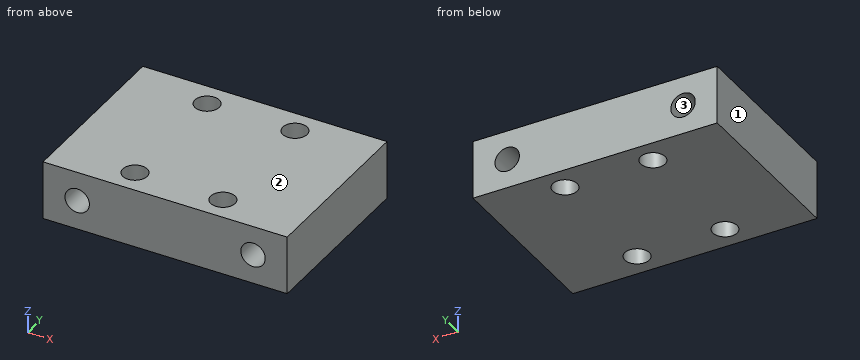
from build123d import *

# Parameters (mm, degrees)
SKETCH_1_W             = 25
SKETCH_1_H             = 18
EXTRUDE_1_DEPTH        = 3
HOLE_WIZARD_M3_1_D     = 2.5
HOLE_WIZARD_M3_2_D     = 2.5
HOLE_WIZARD_M3_2_DEPTH = 8.5
HOLE_WIZARD_M3_2_TIP   = 0.751075774


with BuildPart() as part:
    # 草图1 → 凸台-拉伸1 (new, symmetric)
    with BuildSketch(Plane.XY):
        Rectangle(SKETCH_1_W, SKETCH_1_H)
    extrude(amount=EXTRUDE_1_DEPTH, both=True)

    # M3 螺纹孔1 (through all)
    with Locations(Plane(origin=(0, 9, 0), x_dir=(1, 0, 0), z_dir=(0, 1, 0))):
        with Locations((-9, 0), (9, 0)):
            Hole(HOLE_WIZARD_M3_1_D / 2)

    # M3 螺纹孔2
    with Locations(Plane.XY.offset(3)):
        with Locations((-4.5, -6.5), (4.5, -6.5), (4.5, 6.5), (-4.5, 6.5)):
            Hole(HOLE_WIZARD_M3_2_D / 2, depth=HOLE_WIZARD_M3_2_DEPTH)
            with Locations((0, 0, -(HOLE_WIZARD_M3_2_DEPTH + HOLE_WIZARD_M3_2_TIP / 2))):  # 118° drill point
                Cone(0, HOLE_WIZARD_M3_2_D / 2, HOLE_WIZARD_M3_2_TIP, mode=Mode.SUBTRACT)


solid = part.part
Verification items for the finished model (mm, model axes). Face numbers are marked on the shaded views. Give positions to 0.01 mm unless a question says otherwise; leave off trailing zeros. Write each loop counter-clockwise with the first axis right and the second up, starting at its lowest first coordinate (ties: lowest second). Pieces come first, ordered by that corner, then holes. Notation, with made-up numbers: M 27,61 L 75,61 A14 ccw 75,71 Z; hole C 31.5,58.5 d2. An arc over 180 degrees is marked long. Use CSV: the item, a comma, the result in double quotes.
1) Cross-section at C-C (x = 9). Enter the section's corners in (y, z), plus the area to 3 significant figures.
Final values:
outline,"M -9,-3 L 9,-3 L 9,-1.25 L -9,-1.25 Z; M -9,1.25 L 9,1.25 L 9,3 L -9,3 Z"
area,"63.0 mm²"
2) Cross-section at A-A (y = 6.5). Enter the section's corners in (x, z), plus the area to 3 significant figures.
Final values:
outline,"M -12.5,-3 L -5.75,-3 L -5.75,3 L -12.5,3 Z; M -3.25,-3 L 3.25,-3 L 3.25,3 L -3.25,3 Z; M 5.75,-3 L 12.5,-3 L 12.5,3 L 5.75,3 Z; hole C -9,0 d2.5; hole C 9,0 d2.5"
area,"110 mm²"
3) Cross-section at D-D (y = 2.5). Enter the section's corners in (x, z), plus the area to 3 significant figures.
Final values:
outline,"M -12.5,-3 L 12.5,-3 L 12.5,3 L -12.5,3 Z; hole C -9,0 d2.5; hole C 9,0 d2.5"
area,"140 mm²"
4) Cross-section at B-B (z = -0.75). Enter the section's corners in (x, y), plus the area to 3 significant figures.
Final values:
outline,"M -12.5,-9 L -10,-9 L -10,9 L -12.5,9 Z; M -8,-9 L 8,-9 L 8,9 L -8,9 Z; M 10,-9 L 12.5,-9 L 12.5,9 L 10,9 Z; hole C -4.5,-6.5 d2.5; hole C -4.5,6.5 d2.5; hole C 4.5,-6.5 d2.5; hole C 4.5,6.5 d2.5"
area,"358 mm²"
5) Release check for a two-part mould opening along Z. For the marked faces 1, 2 and 3 record: released by +Z, released by -Z, zero draft, split by the parting line, or undercut.
Final values:
face 1,"zero draft"
face 2,"released by +Z"
face 3,"undercut"
6) Material ranges on line 1 along Y through (x, z) = (-4.5, 0.25); line 2 along X through (y, z) = (-2.25, 0.65); line 3 along X through (y, z) = (-7.5, 0.2), recorded low to high.
Final values:
line 1,"-9 to -7.75, -5.25 to 5.25, 7.75 to 9"
line 2,"-12.5 to -10.07, -7.93 to 7.93, 10.07 to 12.5"
line 3,"-12.5 to -10.23, -7.77 to -5.25, -3.75 to 3.75, 5.25 to 7.77, 10.23 to 12.5"
